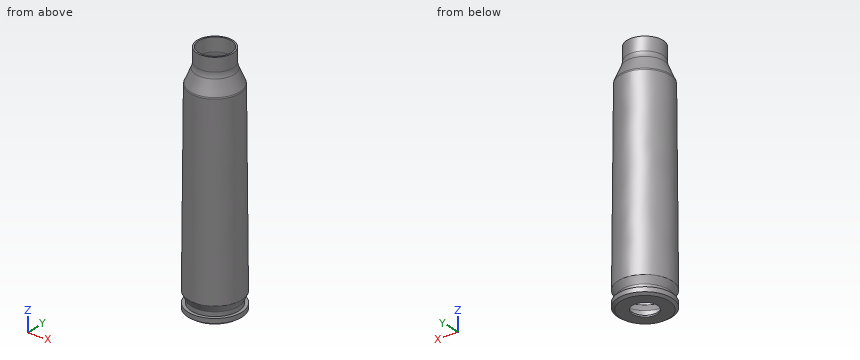
```python
from build123d import *


with BuildPart() as f1:
    # F0 (on Front) → F1 (revolve)
    with BuildSketch(Plane.XZ):
        with BuildLine():
            Line((2.22631, -41.158347), (4.314927, -41.158347))
            Line((4.314927, -41.158347), (4.8, -40.818695))
            Line((4.8, -40.818695), (4.8, -40.013753))
            Line((4.8, -40.013753), (4.215, -40.013753))
            Line((4.215, -40.013753), (4.215, -39.253753))
            Line((4.215, -39.253753), (4.788558, -38.023753))
            Line((4.788558, -38.023753), (4.502255, -4.761092))
            ThreePointArc((4.502255, -4.761092), (4.488875, -4.636308), (4.451402, -4.516533))
            Line((4.451402, -4.516533), (3.416918, -2.079442))
            ThreePointArc((3.416918, -2.079442), (3.265991, -1.593379), (3.215, -1.086984))
            Line((3.215, -1.086984), (3.215, 1.319427))
            Line((3.215, 1.319427), (2.9356, 1.319427))
            Line((2.9356, 1.319427), (2.9356, -1.086984))
            ThreePointArc((2.9356, -1.086984), (2.9922, -1.649082), (3.159729, -2.188612))
            Line((3.159729, -2.188612), (4.194213, -4.625703))
            ThreePointArc((4.194213, -4.625703), (4.215327, -4.693189), (4.222865, -4.763497))
            Line((4.222865, -4.763497), (4.508625, -37.962956))
            Line((4.508625, -37.962956), (3.9356, -39.191812))
            Line((3.9356, -39.191812), (3.9356, -40.293153))
            Line((3.9356, -40.293153), (4.5206, -40.293153))
            Line((4.5206, -40.293153), (4.5206, -40.673249))
            Line((4.5206, -40.673249), (4.226832, -40.878947))
            Line((4.226832, -40.878947), (2.22631, -40.878947))
            Line((2.22631, -40.878947), (2.22631, -41.158347))
        make_face()
    revolve(axis=Axis((0, 0, -19.917163), (0, 0, 1)))


solid = f1.part
```
For this review, take the finished solid that the model builds, in its own axes (mm). Coordinates: 2 decimals unless noted, no trailing zeros. Order: outer loops, then holes, each group sorted by start corner. A loop starts at its lowest first (then second) coordinate and runs counter-clockwise, first axis right, second up. Notation, with made-up numbers: (-32, 57.25) - (16, 57.25) arc R18 cw to (16, 71.25) - close; hole circle Ø7 at (-10.5, -20.5). An arc over 180 degrees is marked (long way). Answer as a JSON object with one key per item and string values. Group by question number.
1. We need section A-A on z = -37.5. State the section outline as (x, y) points, then the cut area to 3 significant figures.
2. We need section B-B on z = -4. State the section outline as (x, y) points, then the cut area to 3 significant figures.
3. Clearance check with flat-ended pins moving along their axes: P1, Ø5.5, axis at x = 0, y = 0, coming from the +Z side; P2, Ø4, axis at x = -1, y = 1.5, coming from the +Z side; P3, Ø2, axis at x = 3, z = -22.5, coming from the +Y side; P4, Ø5, axis at y = -3.5, z = -7.5, coming from the +X side. State where each tip first meets the part, or that it passes through.
4. For probe 1 along Y at (x, z) = (0, 0) (3 decimals); probe 2 along Y at (x, z) = (0, -40.45); probe 3 along Z at (x, y) = (-0.5, -2.75), list the stretches that pass through material, from the lowest coordinate up.
Final values:
{
 "1": {"outline": "circle Ø9.57 at (0, 0); hole circle Ø9.01 at (0, 0)", "area": "8.15 mm²"},
 "2": {"outline": "circle Ø8.46 at (0, 0); hole circle Ø7.86 at (0, 0)", "area": "7.78 mm²"},
 "3": {"P1": "z = -40.88", "P2": "z = 1.32", "P3": "y = 4.2", "P4": "x = 4.41"},
 "4": {"probe 1": "-3.215 to -2.936, 2.936 to 3.215", "probe 2": "-4.8 to -4.52, 4.52 to 4.8", "probe 3": "-41.16 to -40.88"}
}
